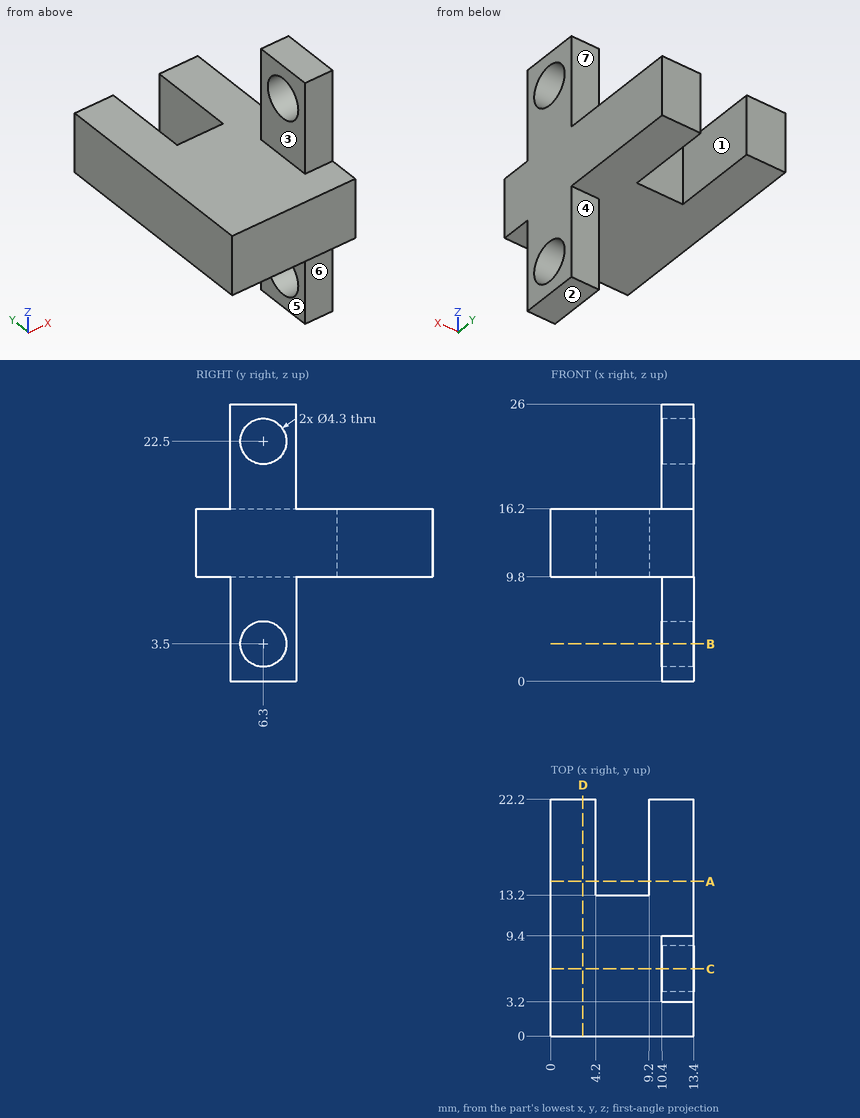
Geometry check sheet. Reference: drawing and pictorial views, mm from the part's lowest x, y, z. A direction names the side the tool comes from. Give positions to 0.01 mm unless a question says otherwise; leave off trailing zeros. Order: outer loops, then holes, each group sorted by start corner. A loop starts at its lowest first (then second) coordinate and runs counter-clockwise, first axis right, second up. Notation, with made-up numbers: M 71,45.5 L 101,45.5 A23 ccw 101,74.5 Z; hole C -18,61.25 d10. An arc over 180 degrees is marked long. Answer in a Markdown table with one row per item. Add a question column.
Q1. Sectioned sample at C-C, the plane y = 6.3. Record the boundary of the cut face in (x, z), and give its area (3 significant figures).
Q2. Sectioned sample at A-A, the plane y = 14.5. Record the boundary of the cut face in (x, z).
Q3. Thickness scan on L1, parallel to Y at x = 11.75, z = 22.5; L2, parallel to Z at x = 1.75, y = 13.25; L3, parallel to Y at x = 11.75, z = 16.75. Record the ranges inside material, lowest first.
Q4. Sectioned sample at D-D, the plane x = 3. Record the boundary of the cut face in (y, z), and give its area (3 significant figures).
Q5. Release check for a two-part mould opening along X. For the marked faces 1, 2 and 3 record: released by +X, released by -X, zero draft, split by the parting line, or undercut.
Q6. Gauge pin test, flat ends, axial feed: pin 1 Ø3.5 at (x, z) = (12.5, 5.5) entering from +Y; pin 2 Ø4 at (x, z) = (7, 14) entering from +Y; pin 3 Ø5 at (y, z) = (5.5, 20.5) entering from -X. Record the tip position at first contact, or that the pin passes through.
Q7. Sectioned sample at B-B, the plane z = 3.5. Record the boundary of the cut face in (x, y), and give its area (3 significant figures).
Q8. Access from +Z, -Z, +X, -X, +Y, -Y to the whole of each face (thin tool, end or side, straight path). Record for the marked faces 4, 5, 6 and 7.
Verdict:
| question | item | result |
|---|---|---|
| 1 | outline | M 0,9.8 L 10.4,9.8 L 10.4,5.65 L 13.4,5.65 L 13.4,20.35 L 10.4,20.35 L 10.4,16.2 L 0,16.2 Z; M 10.4,0 L 13.4,0 L 13.4,1.35 L 10.4,1.35 Z; M 10.4,24.65 L 13.4,24.65 L 13.4,26 L 10.4,26 Z |
| 1 | area | 119 mm² |
| 2 | outline | M 0,9.8 L 4.2,9.8 L 4.2,16.2 L 0,16.2 Z; M 9.2,9.8 L 13.4,9.8 L 13.4,16.2 L 9.2,16.2 Z |
| 3 | L1 | 3.2 to 4.15, 8.45 to 9.4 |
| 3 | L2 | 9.8 to 16.2 |
| 3 | L3 | 3.2 to 9.4 |
| 4 | outline | M 0,9.8 L 22.2,9.8 L 22.2,16.2 L 0,16.2 Z |
| 4 | area | 142 mm² |
| 5 | face 1 | undercut |
| 5 | face 2 | zero draft |
| 5 | face 3 | released by -X |
| 6 | pin 1 | y = 9.4 |
| 6 | pin 2 | y = 13.2 |
| 6 | pin 3 | x = 10.4 |
| 7 | outline | M 10.4,3.2 L 13.4,3.2 L 13.4,4.15 L 10.4,4.15 Z; M 10.4,8.45 L 13.4,8.45 L 13.4,9.4 L 10.4,9.4 Z |
| 7 | area | 5.70 mm² |
| 8 | face 4 | -Z, +X, -X, +Y |
| 8 | face 5 | -Z, -X, +Y, -Y |
| 8 | face 6 | -Z, +X, -X, -Y |
| 8 | face 7 | +Z, +X, -X, +Y |
